Read the model definition and answer for the solid it produces. Units are mm, in the model's axes. A direction names the side the tool comes from. Round coordinates to 2 decimals unless told otherwise and drop trailing zeros. Write each loop counter-clockwise with the first axis right and the second up, starting at its lowest first coordinate (ties: lowest second). Pieces come first, ordered by that corner, then holes. Notation, with made-up numbers: (23.5, 62) -> (65.5, 62) arc R24 ccw to (65.5, 94) -> close; hole circle Ø10 at (58.5, 26). An arc over 180 degrees is marked (long way). Return JSON: item names as keys, results as strings. Group by question number.
(1) A cutting plane is placed at C-C on y = 0.45. Give the vertices of the cut face in (x, z), then the cut area to 3 significant figures.
(2) The mould has two halves that part along X. Classify faces 1 (the flat face through (5, 1, 20.034)), 2 (the cylindrical face through (1.225, 0.74, -25.296)), 3 (the flat face through (16.9, 1, -13)): released by +X, released by -X, zero draft, split by the parting line, or undercut.
(3) A cutting plane is placed at B-B on x = 6.5. Give the vertices of the cut face in (y, z).
(4) For faces 4 (the flat face through (13, 1, -45.966)), 5 (the flat face through (11, 0, -15)), determine the directions among +Z, -Z, +X, -X, +Y, -Y from which every point of the face is accessible in a straight line to the end or side of a thin tool.
(5) A cutting plane is placed at A-A on z = -14. Give the vertices of the cut face in (x, y).
(6) A cutting plane is placed at D-D on z = -41.5. Give the vertices of the cut face in (x, y), then the cut area to 3 significant figures.
(7) Straight lines are drawn through the part: line 1 (X direction, y = 0.9, z = -18.5); line 2 (Z direction, x = -2, y = 0.7); line 3 (Z direction, x = 15.5, y = 0.15). For each, find the intervals that lie inside material, in ascending order.
(8) Given pin 1 (0.8 mm diameter, centred on y = 1, z = -47, fed in from +X), flat-ended and moving along its own axis, determine where the tip first touches the part or whether it passes through.
Autodesk Inventor part; units mm, degrees
ref_plane "YZ Plane" through (0, 0, 0) normal (1, 0, 0) x (0, 1, 0)
ref_plane "XZ Plane" through (0, 0, 0) normal (0, 1, 0) x (-1, 0, 0)
ref_plane "XY Plane" through (0, 0, 0) normal (0, 0, 1) x (1, 0, 0)
sketch "Sketch1" plane through (0, 0, 0) normal (0, 1, 0) x (-1, 0, 0)
  line L0 (4.5998, 20.0337) -> (-14.9002, 20.0337)
  line L1 (6.3706, -32.4029) -> (-3.3383, -50.8959)
  line L2 (6.5998, -31.4732) -> (6.5998, 18.0337)
  line L3 (-5.1091, -51.9663) -> (-14.9002, -51.9663)
  circle A0 centre (1.5998, 15.0337) radius 2.5
  circle A1 centre (-5.4002, -18.9663) radius 6
  line L4 (-14.9002, -45.9663) -> (-12.597, -45.9663)
  line L5 (-12.0688, -48.9663) -> (-14.0688, -48.9663)
  line L6 (-16.9002, 18.0337) -> (-16.9002, -43.9663)
  arc A2 (-16.9002, -43.9663) -> (-14.9002, -45.9663) centre (-14.9002, -43.9663) ccw
  arc A3 (-5.1091, -51.9663) -> (-3.3383, -50.8959) centre (-5.1091, -49.9663) ccw
  arc A4 (6.3706, -32.4029) -> (6.5998, -31.4732) centre (4.5998, -31.4732) ccw
  arc A5 (6.5998, 18.0337) -> (4.5998, 20.0337) centre (4.5998, 18.0337) ccw
  arc A6 (-14.9002, 20.0337) -> (-16.9002, 18.0337) centre (-14.9002, 18.0337) ccw
  circle A7 centre (-14.4002, -18.9663) radius 1.5
  circle A8 centre (-0.9002, -11.172) radius 1.5
  circle A9 centre (-0.9002, -26.7605) radius 1.5
  line L7 (-12.597, -45.9663) -> (-11.9002, -45.9663)
  line L8 (-10.9002, -46.9663) -> (-10.9002, -47.9663)
  line L9 (-12.3368, -48.9663) -> (-11.9002, -48.9663)
  line L10 (-14.9002, -51.9663) -> (-15.9002, -51.9663)
  line L11 (-16.9002, -50.9663) -> (-16.9002, -49.9663)
  line L12 (-15.9002, -48.9663) -> (-14.0688, -48.9663)
  arc A10 (-10.9002, -46.9663) -> (-11.9002, -45.9663) centre (-11.9002, -46.9663) ccw
  arc A11 (-11.9002, -48.9663) -> (-10.9002, -47.9663) centre (-11.9002, -47.9663) ccw
  arc A12 (-15.9002, -48.9663) -> (-16.9002, -49.9663) centre (-15.9002, -49.9663) ccw
  arc A13 (-16.9002, -50.9663) -> (-15.9002, -51.9663) centre (-15.9002, -50.9663) ccw
  point P0 (0, 0)
  point P1 (6.5998, 20.0337)
  point P2 (-16.9002, 20.0337)
  point P3 (6.5998, -31.9663)
  point P4 (-3.9002, -51.9663)
  point P5 (-16.9002, -45.9663)
  point P6 (-10.9002, -45.9663)
  point P7 (-10.9002, -48.9663)
  point P8 (-16.9002, -51.9663)
  point P9 (-16.9002, -48.9663)
  dimension "d1" = 23.5
  dimension "d3" = 52
  dimension "d5" = 5
  dimension "d6" = 5
  dimension "d7" = 5
  dimension "d8" = 12
  dimension "d9" = 12
  dimension "d10" = 39
  dimension "d28" = 3
  dimension "d29" = 9
  dimension "d30" = 2.5
  dimension "d31" = 3
  dimension "d32" = 3
  dimension "d33" = 120
  dimension "d34" = 120
  dimension "d35" = 9
  dimension "d36" = 9
  dimension "d37" = 3
  dimension "d38" = 6
  dimension "d39" = 3
  dimension "d40" = 6
  dimension "d41" = 1
  dimension "d44" = 13
extrude "Extrusion1" add sketch "Sketch1" along normal blind 1.5
properties part number "bras_amortisseur"
Checks:
{
 "1": {"outline": "(-6.6, -31.47) arc R2 ccw to (-6.37, -32.4) -> (3.34, -50.9) arc R2 ccw to (5.11, -51.97) -> (15.9, -51.97) arc R1 ccw to (16.9, -50.97) -> (16.9, -49.97) arc R1 ccw to (15.9, -48.97) -> (11.9, -48.97) arc R1 cw to (10.9, -47.97) -> (10.9, -46.97) arc R1 cw to (11.9, -45.97) -> (14.9, -45.97) arc R2 ccw to (16.9, -43.97) -> (16.9, 18.03) arc R2 ccw to (14.9, 20.03) -> (-4.6, 20.03) arc R2 ccw to (-6.6, 18.03) -> close; hole circle Ø5 at (-1.6, 15.03); hole circle Ø3 at (0.9, -26.76); hole circle Ø12 at (5.4, -18.97); hole circle Ø3 at (0.9, -11.17); hole circle Ø3 at (14.4, -18.97)", "area": "1,410 mm^2"},
 "2": {"face 1": "zero draft", "face 2": "undercut", "face 3": "released by +X"},
 "3": {"outline": "(0, -51.97) -> (1.5, -51.97) -> (1.5, -24.86) -> (0, -24.86) -> close; (0, -13.07) -> (1.5, -13.07) -> (1.5, 20.03) -> (0, 20.03) -> close"},
 "4": {"face 4": "+X, +Y, -Y", "face 5": "+Z, -Z, +X, -X, -Y"},
 "5": {"outline": "(-6.6, 0) -> (2.03, 0) -> (2.03, 1.5) -> (-6.6, 1.5) -> close; (8.77, 0) -> (16.9, 0) -> (16.9, 1.5) -> (8.77, 1.5) -> close"},
 "6": {"outline": "(-1.59, 0) -> (16.9, 0) -> (16.9, 1.5) -> (-1.59, 1.5) -> close", "area": "27.7 mm^2"},
 "7": {"line 1": "x = -6.6 to -0.58, 11.38 to 12.97, 15.83 to 16.9", "line 2": "z = -40.73 to 12.57, 17.5 to 20.03", "line 3": "z = -51.97 to -48.97, -45.87 to -19.99, -17.95 to 19.94"},
 "8": {"pin 1": "stops at x = 10.97"}
}
